Work out the finished part from the listing and answer in its coordinate system (mm). A direction names the side the tool comes from. Give positions to 0.01 mm unless a question says otherwise; leave off trailing zeros. Loops run counter-clockwise (first coordinate to the right, second up) from the corner with the lowest first, then second, coordinate; pieces in that order, holes last. Notation, with made-up numbers: M 85,-27.5 L 100,-27.5 A24 ccw 100,-12.5 Z; hole C 19,45 d10. An arc over 180 degrees is marked long. Answer in a Markdown table with one row per item. Add a question column.
from build123d import *

# Parameters (mm, degrees)
F2_R     = 10
F3_DEPTH = 25.0000003725
F4_T     = -2.5


with BuildPart() as f1:
    # F0 (on Front) → F1 (revolve)
    with BuildSketch(Plane.XZ):
        with BuildLine():
            Line((0, 35), (0, 0))
            Line((0, 0), (85, 0))
            ThreePointArc((85, 0), (75.9723603269, 23.5370065806), (53.520439725, 35))
            Line((53.520439725, 35), (0, 35))
        make_face()
    revolve(axis=Axis((0, 0, 17.5), (0, 0, -1)))

    # F2 (on face) → F3 (cut)
    with BuildSketch(Plane.XY.offset(35)):
        with Locations((7.7254248594, 23.7764129074)):
            Circle(F2_R)
        with Locations((25, 0)):
            Circle(F2_R)
        with Locations((7.7254248594, -23.7764129074)):
            Circle(F2_R)
        with Locations((-20.2254248594, 14.6946313073)):
            Circle(F2_R)
    extrude(amount=-F3_DEPTH, mode=Mode.SUBTRACT)

    # F4
    f4_openings = [f1.faces().sort_by_distance(p)[0] for p in [
        (0, 0, 0),
    ]]
    offset(amount=F4_T, openings=f4_openings, kind=Kind.INTERSECTION)

    # F5 (on Right) → F6 (revolve, cut)
    with BuildSketch(Plane.YZ):
        Polygon((40.5379161239, 62.8329962492), (0, 62.8329962492), (0, 0), align=None)
    revolve(axis=Axis((0, 0, 31.4164981246), (0, 0, 1)), mode=Mode.SUBTRACT)


solid = f1.part
(1) The mould has two halves that part along X. Classify faces 1 (the face through (23, 11, 35)), 2 (the face through (-20, 15, 10)): pulls with the +X half, pulls with the -X half, needs draft (parallel to the pull), parting line crosses it, or undercut.
(2) Consider line 1 along X through (y, z) = (30, 27.5); line 2 along Y through (x, z) = (4.5, 28.5); line 3 along X through (y, z) = (7, 23). Determine where each line is inside the solid, lowest interval first. Write a range as from..to.
(3) Section B-B, the plane x = 0 is taken. Determine the outline of the cut face in (y, z).
(4) Section A-A, the plane z = 17 is taken. State how many separate pieces and enclosed holes the cut face has, and give its area (3 significant figures).
(5) Each of these flat-tipped pins is pushed along its axis until it touches: P1, Ø7.5, axis at x = 19, y = 4.5, coming from the -Z side; P2, Ø12, axis at x = 62, z = 12, coming from the +Y side; P3, Ø3, axis at x = 28, z = 19.5, coming from the +Y side. Where does it stop, or does it pass through?
(6) Which of the six approach directions +Z, -Z, +X, -X, +Y, -Y give full straight-line access (tool end or side, diameter ignored) to faces 3 (the face through (44, -70, 0)), 4 (the face through (36.923, 3.755, 20.175)), 5 (the face through (8, 24, 10))?
Numbers:
| question | item | result |
|---|---|---|
| 1 | face 1 | needs draft |
| 1 | face 2 | undercut |
| 2 | line 1 | x = -65.2..-60.46, -3.12..-0.1, 15.55..18.57, 60.46..65.2 |
| 2 | line 2 | y = -70.31..-65.68, -35.85..-33.24, 33.24..35.85, 65.68..70.31 |
| 2 | line 3 | x = -76.12..-72.71, -30.08..-26.61, -13.84..-13.08, 14.64..17.86, 32.14..35.36, 72.71..76.12 |
| 3 | outline | M -85,0 L -82.5,0 A32.7 cw -53.39,32.5 L -33.6,32.5 L -33.6,7.5 L -13.95,7.5 L -13.95,21.62 L -17.43,27.01 L -17.43,10 L -30.13,10 L -30.13,35 L -53.52,35 A35.2 ccw Z; M 13.95,7.5 L 33.6,7.5 L 33.6,32.5 L 53.39,32.5 A32.7 cw 82.5,0 L 85,0 A35.2 ccw 53.52,35 L 30.13,35 L 30.13,10 L 17.43,10 L 17.43,27.01 L 13.95,21.62 Z |
| 4 | separate pieces | 5 |
| 4 | enclosed holes | 5 |
| 4 | area | 2,140 mm² |
| 5 | P1 | stops at z = 7.5 |
| 5 | P2 | stops at y = 61.71 |
| 5 | P3 | stops at y = 75.14 |
| 6 | face 3 | -Z, +X, -X, +Y, -Y |
| 6 | face 4 | -Z |
| 6 | face 5 | +Z |
